Could you check a few things on this model? Use its own coordinates, in mm. Face numbers are marked on the shaded views. A direction names the side the tool comes from. Round coordinates to 2 decimals unless told otherwise and drop trailing zeros. One line per item, written item: value.
```python
from build123d import *

# Parameters (mm, degrees)
SKETCH2_R           = 5.5
SKETCH2_R_2         = 1
BOSS_EXTRUDE1_DEPTH = 10
SKETCH3_R           = 2.8
CUT_EXTRUDE1_DEPTH  = 3
SKETCH4_R           = 1.42
CUT_EXTRUDE2_DEPTH  = 7
SKETCH5_R           = 22.131734032
SKETCH5_R_2         = 10
CUT_EXTRUDE3_DEPTH  = 10


with BuildPart() as part:
    # Sketch1 → Revolve1 (revolve)
    with BuildSketch(Plane.XY, mode=Mode.PRIVATE) as revolve1_sk:
        with BuildLine():
            Line((-7, 9), (5, 9))
            add(Edge.make_bspline(
                [(5, 9), (5, 8.856466181), (4.980630385, 8.552638111), (4.879856885, 8.085906437), (4.637540593, 7.528306389), (3.996049584, 6.69016035), (2.86097235, 5.618747783), (1.478465211, 4.503997435), (0.514957064, 3.794701588), (0.068439653, 3.476275963), (0, 3.427716912)],
                knots=[0, 0, 0, 0, 0.0625, 0.125, 0.25, 0.375, 0.5, 0.625, 0.75, 0.773497894, 0.773497894, 0.773497894, 0.773497894], degree=3))
            Line((0, 3.427716912), (0, 1))
            add(Edge.make_bspline(
                [(7, 9), (7, 7.437991686), (5.451200792, 4.581787455), (0.00160793, 1.001387392), (0, 1)],
                knots=[0, 0, 0, 0, 0.405901642, 1, 1, 1, 1], degree=3))
            Line((7, 9), (7, 11))
            Line((7, 11), (6, 11))
            Line((6, 11), (6, 10.9))
            ThreePointArc((6, 10.9), (5.736396103, 10.263603897), (5.1, 10))
            Line((5.1, 10), (-5.1, 10))
            ThreePointArc((-5.1, 10), (-5.736396103, 10.263603897), (-6, 10.9))
            Line((-6, 10.9), (-6, 11))
            Line((-6, 11), (-7, 11))
            Line((-7, 11), (-7, 9))
        make_face()
    revolve(revolve1_sk.sketch.rotate(Axis((0, 0, 0), (1, 0, 0)), 90), axis=Axis((0, 0, 0), (1, 0, 0)))

    # Sketch2 → Boss-Extrude1 (add)
    with BuildSketch(Plane.ZY.offset(7)):
        Circle(SKETCH2_R)
        Circle(SKETCH2_R_2, mode=Mode.SUBTRACT)
    extrude(amount=-BOSS_EXTRUDE1_DEPTH)

    # Sketch3 → Cut-Extrude1 (cut)
    with BuildSketch(Plane(origin=(3, 0, 0), x_dir=(0, 0, -1), z_dir=(1, 0, 0))):
        Circle(SKETCH3_R)
    extrude(amount=-CUT_EXTRUDE1_DEPTH, mode=Mode.SUBTRACT)

    # Sketch4 → Cut-Extrude2 (cut)
    with BuildSketch(Plane.ZY.offset(7)):
        Circle(SKETCH4_R)
    extrude(amount=-CUT_EXTRUDE2_DEPTH, mode=Mode.SUBTRACT)

    # Sketch5 → Cut-Extrude3 (cut)
    with BuildSketch(Plane(origin=(0, 0, 0), x_dir=(0, 0, -1), z_dir=(1, 0, 0))):
        Circle(SKETCH5_R)
        with Locations(Location((0, 0, 0), (0, 0, 180))):
            Circle(SKETCH5_R_2, mode=Mode.SUBTRACT)
    extrude(amount=-CUT_EXTRUDE3_DEPTH, mode=Mode.SUBTRACT)


solid = part.part
```
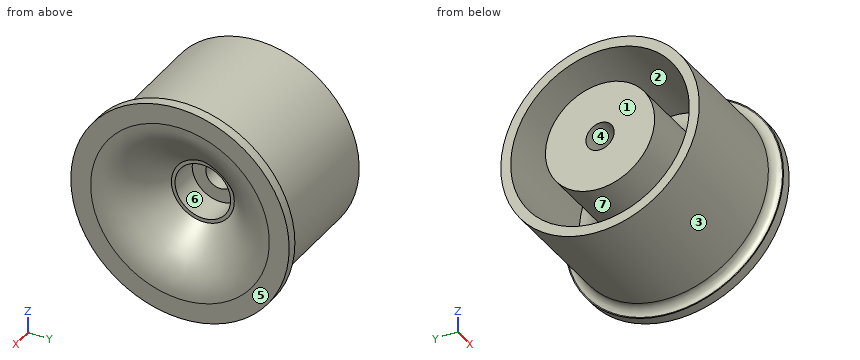
(1) On a 3-axis mill with a long thin cutter (end or side, diameter ignored), from which of +Z, -Z, +X, -X, +Y, -Y can I reach the whole of each face in a straight line? I mean the marked faces 5, 6 and 7. Say none if no direction works.
Results below:
face 5: +Z, -Z, +X, +Y, -Y
face 6: +X
face 7: -X
(2) We'd pull the mould along Y, two halves only. Please class the marked faces 1, 2, 3 and 4: +Y half, -Y half, draft (parallel to the pull), parting line (faces both ways), or undercut.
Results below:
face 1: draft
face 2: undercut
face 3: parting line
face 4: undercut
(3) For pin 1 Ø4.5 at (y, z) = (0, 0) entering from +X; pin 2 Ø7.5 at (y, z) = (0, 0) entering from +X; pin 3 Ø2 at (x, y) = (3.5, 8) entering from +Z, each with a flat end and sliding along its axis, tell me the tip position at first contact or that it passes through.
Results below:
pin 1: stops at x = 0
pin 2: stops at x = 3.72
pin 3: stops at z = 7.14
(4) Imagine slicing it at A-A on x = 4.5. Give the number of separate pieces and of enclosed holes in the cut face, then the cut area to 3 significant figures.
Results below:
separate pieces: 2
enclosed holes: 2
area: 169 mm²
(5) Please list where these lines run through material, in increasing order: L1, parallel to Y at x = -1.25, z = 0; L2, parallel to Z at x = -4.25, y = -3.5; L3, parallel to Y at x = -2.5, z = 0.5.
Results below:
L1: y = -10 to -9, -5.5 to -1.42, 1.42 to 5.5, 9 to 10
L2: z = -9.37 to -8.29, -4.24 to 4.24, 8.29 to 9.37
L3: y = -9.99 to -8.99, -5.48 to -1.33, 1.33 to 5.48, 8.99 to 9.99
